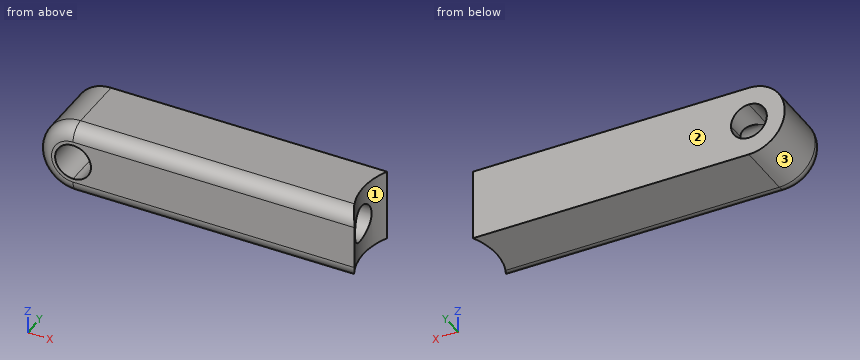
from build123d import *

# Parameters (mm, degrees)
F1_DEPTH = 12.7
F2_R     = 2.54
F3_R     = 3.175
F4_DEPTH = 50.8
F5_R     = 12.7
F6_DEPTH = 38.1


with BuildPart() as f1:
    # F0 (on Front) → F1 (new body)
    with BuildSketch(Plane.XZ):
        with BuildLine():
            ThreePointArc((-50.8, -6.35), (-46.3098719395, -4.4901280605), (-44.45, 0))
            ThreePointArc((-44.45, 0), (-46.3098719395, 4.4901280605), (-50.8, 6.35))
            Line((-50.8, 6.35), (-50.8, 3.175))
            ThreePointArc((-50.8, 3.175), (-48.5549359697, 2.2450640303), (-47.625, 0))
            ThreePointArc((-47.625, 0), (-48.5549359697, -2.2450640303), (-50.8, -3.175))
            Line((-50.8, -3.175), (-50.8, -6.35))
        make_face()
        with BuildLine():
            ThreePointArc((-50.8, 6.35), (-46.3098719395, 4.4901280605), (-44.45, 0))
            ThreePointArc((-44.45, 0), (-46.3098719395, -4.4901280605), (-50.8, -6.35))
            Line((-50.8, -6.35), (0, -6.35))
            Line((0, -6.35), (0, 6.35))
            Line((0, 6.35), (-50.8, 6.35))
        make_face()
        with BuildLine():
            Line((-50.8, 3.175), (-50.8, 6.35))
            ThreePointArc((-50.8, 6.35), (-57.15, 0), (-50.8, -6.35))
            Line((-50.8, -6.35), (-50.8, -3.175))
            ThreePointArc((-50.8, -3.175), (-53.975, 0), (-50.8, 3.175))
        make_face()
    extrude(amount=F1_DEPTH)

    # F2
    f2_edges = [f1.edges().sort_by_distance(p)[0] for p in [
        (-25.4, -12.7, -6.35),
    ]]
    fillet(f2_edges, radius=F2_R)

    # F3 (on Right) → F4 (cut, symmetric)
    with BuildSketch(Plane.YZ):
        with Locations((-6.35, 0)):
            Circle(F3_R)
    extrude(amount=F4_DEPTH, both=True, mode=Mode.SUBTRACT)

    # F5 (on Top) → F6 (cut, symmetric)
    with BuildSketch(Plane.XY):
        with Locations((9.5227770507, -5.5082733743)):
            Circle(F5_R)
    extrude(amount=F6_DEPTH, both=True, mode=Mode.SUBTRACT)


solid = f1.part
The model under review builds one solid part; all positions refer to its coordinate system, in mm. Face numbers are marked on the shaded views. Round coordinates to 2 decimals unless told otherwise and drop trailing zeros. Loops run counter-clockwise (first coordinate to the right, second up) from the corner with the lowest first, then second, coordinate; pieces in that order, holes last. Notation, with made-up numbers: (0, 57) -> (19, 57) arc R19 cw to (19, 94) -> close; hole circle Ø2 at (-6, -36). An arc over 180 degrees is marked (long way). Answer as CSV lines item,"result".
1) For P1, Ø1, axis at y = -5.5, z = 3.5, coming from the -X side; P2, Ø5, axis at y = -6.35, z = 0, coming from the +X side, all flat-tipped, find the tip position at first contact; note any pin that passes through.
Geometry results:
P1,"stops at x = -56.4"
P2,"stops at x = -52.76"
2) Add section B-B on y = -11.25. Write out the cut boundary in (x, z) (3 decimals), plus the area to 3 significant figures.
Geometry results:
outline,"(-50.8, -6.104) -> (-1.805, -6.104) -> (-1.805, 6.104) -> (-50.8, 6.104) arc R6.104 ccw to start; hole circle Ø6.35 at (-50.8, 0)"
area,"625 mm²"
3) To check wall thickness, follow line 1 along Z through (x, y) = (-37, -6.35) (3 decimals); line 2 along Y through (x, z) = (-39.5, 0) (3 decimals); line 3 along Z through (x, y) = (-39, -4.75). State the ranges of each line that lie inside material, in increasing order. Write a range as from..to.
Geometry results:
line 1,"z = -6.35..-3.175, 3.175..6.35"
line 2,"y = -12.7..-9.525, -3.175..0"
line 3,"z = -6.35..-2.74, 2.74..6.35"
4) Add section A-A on x = -34. Write out the cut boundary in (y, z) (3 decimals).
Geometry results:
outline,"(-12.7, -3.81) arc R2.54 ccw to (-10.16, -6.35) -> (0, -6.35) -> (0, 6.35) -> (-10.16, 6.35) arc R2.54 ccw to (-12.7, 3.81) -> close; hole circle Ø6.35 at (-6.35, 0)"
5) Draft analysis for pull direction Y (two halves, no side actions). For the marked faces 1, 2 and 3, state which applies: pulls with the +Y half, pulls with the -Y half, needs draft (parallel to the pull), parting line crosses it, or undercut.
Geometry results:
face 1,"undercut"
face 2,"pulls with the +Y half"
face 3,"needs draft"
6) Add section D-D on y = -5.5. Write out the cut boundary in (x, z) (3 decimals).
Geometry results:
outline,"(-50.8, -6.35) -> (-3.177, -6.35) -> (-3.177, -3.059) -> (-49.95, -3.059) arc R3.175 cw (long way) to (-49.95, 3.059) -> (-3.177, 3.059) -> (-3.177, 6.35) -> (-50.8, 6.35) arc R6.35 ccw to start"
7) Add section C-C on x = -49. Write out the cut boundary in (y, z) (3 decimals).
Geometry results:
outline,"(-12.7, -3.81) arc R2.54 ccw to (-10.16, -6.35) -> (0, -6.35) -> (0, -2.615) -> (-4.55, -2.615) arc R3.175 cw to (-8.15, -2.615) -> (-12.7, -2.615) -> close; (-12.7, 2.615) -> (-8.15, 2.615) arc R3.175 cw to (-4.55, 2.615) -> (0, 2.615) -> (0, 6.35) -> (-10.16, 6.35) arc R2.54 ccw to (-12.7, 3.81) -> close"
